The listing builds one solid part. Answer for the finished solid, in the listing's coordinates (mm). Give positions to 0.01 mm unless a question says otherwise; leave off trailing zeros. Write each loop counter-clockwise with the first axis right and the second up, starting at its lowest first coordinate (ties: lowest second). Pieces come first, ordered by that corner, then holes. Notation, with made-up numbers: M -9.75,-17 L 2.25,-17 A22 ccw 2.25,-3 Z; hole C 65.25,60.25 d6. An arc over 180 degrees is marked long. Return JSON: item names as keys, results as strings.
from build123d import *

# Parameters (mm, degrees)
SKETCH1_R           = 6
SKETCH1_R_2         = 4
BOSS_EXTRUDE1_DEPTH = 2.9


with BuildPart() as part:
    # Sketch1 → Boss-Extrude1 (new body)
    with BuildSketch(Plane.XY.offset(-137.9)):
        Polygon((118.9, 2.9), (100, 2.9), (100, 0.5), (99.5, 0), (70.5, 0), (70, 0.5), (70, 2.9), (15, 2.9), (15, 0.5), (14.5, 0), (-14.5, 0), (-15, 0.5), (-15, 2.9), (-55, 2.9), (-55, 0.5), (-55.5, 0), (-84.5, 0), (-85, 0.5), (-85, 2.9), (-118.9, 2.9), (-118.9, 18.675), (-116, 18.675), (-116, 34.525), (-118.9, 34.525), (-118.9, 50.275), (-116, 50.275), (-116, 66.125), (-118.9, 66.125), (-118.9, 81.9), (-85, 81.9), (-85, 84.3), (-84.5, 84.8), (-55.5, 84.8), (-55, 84.3), (-55, 81.9), (70, 81.9), (70, 84.3), (70.5, 84.8), (99.5, 84.8), (100, 84.3), (100, 81.9), (118.9, 81.9), (118.9, 66.125), (116, 66.125), (116, 50.275), (118.9, 50.275), (118.9, 34.525), (116, 34.525), (116, 18.675), (118.9, 18.675), align=None)
        with Locations((-90.5, 45)):
            Circle(SKETCH1_R, mode=Mode.SUBTRACT)
        with Locations((-38, 45)):
            Circle(SKETCH1_R_2, mode=Mode.SUBTRACT)
    extrude(amount=BOSS_EXTRUDE1_DEPTH)


solid = part.part
Item 1: A cutting plane is placed at A-A, the plane x = -90.5. Write down the section's boundary in (y, z).
Geometry results:
{"outline": "M 2.9,-137.9 L 39,-137.9 L 39,-135 L 2.9,-135 Z; M 51,-137.9 L 81.9,-137.9 L 81.9,-135 L 51,-135 Z"}
Item 2: Given pin 1 Ø1.5 at (x, z) = (-16, -136.5) entering from +Y; pin 2 Ø19 at (x, y) = (-90.5, 45) entering from -Z; pin 3 Ø0.7 at (y, z) = (82.5, -137) entering from +X; pin 4 Ø1.5 at (y, z) = (61, -136) entering from -X, each flat-ended and moving along its own axis, determine where each tip first touches the part or whether it passes through.
Geometry results:
{"pin 1": "stops at y = 81.9", "pin 2": "stops at z = -137.9", "pin 3": "stops at x = 100", "pin 4": "stops at x = -116"}
Item 3: Find the intervals of material crossed by line 1 (Y direction, x = -90.5, z = -135.75); line 2 (Y direction, x = -38, z = -136.7); line 3 (X direction, y = 66, z = -135.65), in increasing order.
Geometry results:
{"line 1": "y = 2.9 to 39, 51 to 81.9", "line 2": "y = 2.9 to 41, 49 to 81.9", "line 3": "x = -116 to 116"}
Item 4: A cutting plane is placed at D-D, the plane x = -38. Write down the section's boundary in (y, z).
Geometry results:
{"outline": "M 2.9,-137.9 L 41,-137.9 L 41,-135 L 2.9,-135 Z; M 49,-137.9 L 81.9,-137.9 L 81.9,-135 L 49,-135 Z"}
Item 5: A cutting plane is placed at C-C, the plane z = -136.3. Count the separate pieces of the cut face and the enclosed holes in it, plus the area to 3 significant figures.
Geometry results:
{"separate pieces": "1", "enclosed holes": "2", "area": "18,900 mm2"}
Item 6: Determine the mould class of faces 1 (the flat face through (2, 43, -135)), 2 (the cylindrical face through (-96.494, 45.264, -136.47)), 3 (the cylindrical face through (-41.2, 42.6, -136.5)) for opening direction Y: +Y half, -Y half, draft (parallel to the pull), parting line (faces both ways), or undercut.
Geometry results:
{"face 1": "draft", "face 2": "undercut", "face 3": "undercut"}
Item 7: A cutting plane is placed at B-B, the plane y = 45. Write down the section's boundary in (x, z).
Geometry results:
{"outline": "M -118.9,-137.9 L -96.5,-137.9 L -96.5,-135 L -118.9,-135 Z; M -84.5,-137.9 L -42,-137.9 L -42,-135 L -84.5,-135 Z; M -34,-137.9 L 118.9,-137.9 L 118.9,-135 L -34,-135 Z"}
